Design review of the part built by this model. Coordinates are the model's own, in mm. Face numbers are marked on the shaded views. A direction names the side the tool comes from. Give positions to 0.01 mm unless a question says otherwise; leave off trailing zeros. Loops run counter-clockwise (first coordinate to the right, second up) from the corner with the lowest first, then second, coordinate; pieces in that order, holes last. Notation, with made-up numbers: (70, -1) -> (108, -1) arc R19 cw to (108, 34) -> close; hole circle Ø11 at (45, 60). An arc over 180 degrees is marked (long way). Use CSV: the item, a comma, the result in double quotes. Start each with the question number.
Item 1: We need section A-A (z = -52). State the section outline as (x, y) points, plus the area to 3 significant figures.
Item 2: Wall thickness on line 1 along Z through (x, y) = (23.5, -53); line 2 along Z through (x, y) = (13, 28.5); line 3 along Y through (x, z) = (16.75, -2.5): over which ranges is each line inside the solid? List them lowest first. Write a range as from..to.
Item 3: The part is to be moulded in two halves that separate along Z. For the marked faces 1, 2 and 3, say which applies: +Z half, -Z half, draft (parallel to the pull), parting line (faces both ways), or undercut.
Item 4: We need section B-B (y = 41.91). State the section outline as (x, z) points, plus the area to 3 significant figures.
Item 5: We need section D-D (x = 14.5). Count the separate pieces of the cut face and the enclosed holes in it, plus the area to 3 significant figures.
Item 6: We need section C-C (y = -29). State the section outline as (x, z) points, plus the area to 3 significant figures.
Item 7: Clearance check with flat-ended pins moving along their axes: pin 1 (5 mm diameter, centred on x = 8.5, y = 10, fed in from +Z); pin 2 (3 mm diameter, centred on y = -64.5, z = 6, fed in from -X); pin 3 (16.5 mm diameter, centred on y = -51.14, z = -30.23, fed in from +X); pin 4 (17 mm diameter, centred on y = -9.525, z = 0, fed in from +X). State where each tip first meets the part, or that it passes through.
Item 8: For the marked faces 4 and 5, list the 3-axis set-ups (+Z, -Z, +X, -X, +Y, -Y) from which the entire face can be reached by the end or side of a thin tool; tool diameter is ignored.
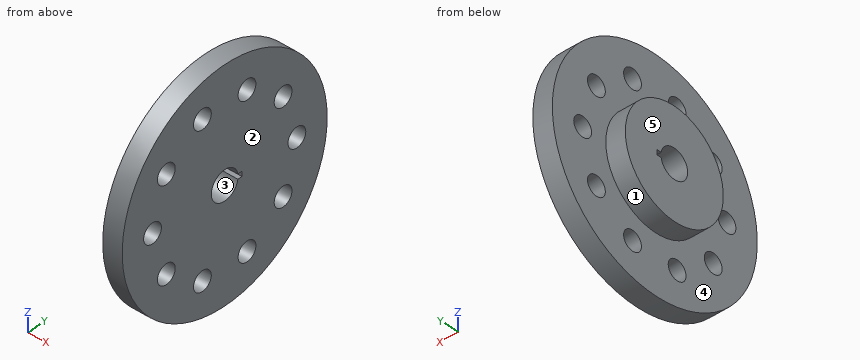
Autodesk Inventor part; units mm, degrees
ref_plane "YZ Plane" through (0, 0, 0) normal (1, 0, 0) x (0, 1, 0)
ref_plane "XZ Plane" through (0, 0, 0) normal (0, 1, 0) x (-1, 0, 0)
ref_plane "XY Plane" through (0, 0, 0) normal (0, 0, 1) x (1, 0, 0)
sketch "Sketch1" plane through (0, 0, 0) normal (0, 0, 1) x (1, 0, 0)
  line L0 (0, 0) -> (0, 25.4)
  line L1 (0, 25.4) -> (12.7, 25.4)
  line L2 (12.7, 25.4) -> (12.7, 63.5)
  line L3 (12.7, 63.5) -> (25.4, 63.5)
  line L4 (25.4, 63.5) -> (25.4, 0)
  line L5 (25.4, 0) -> (0, 0)
  line L6 (0, -9.525) -> (25.4, -9.525)
  dimension "d0" = 25.4
  dimension "d1" = 63.5
  dimension "d2" = 12.7
  dimension "d3" = 25.4
  dimension "d4" = 9.525
revolve "Revolution1" add sketch "Sketch1" angle 360 about axis through (0, -9.525, 0) along (1, 0, 0)
sketch "Sketch2" plane through (12.7, -9.525, 0) normal (-1, 0, 0) x (0, 0, 1)
  circle A0 centre (0, 0) radius 51.435 construction
  circle A1 centre (0, 0) radius 9.525
  circle A2 centre (0, 0) radius 73.025
  circle A3 centre (0, 0) radius 34.925
  point P0 (0, 9.525)
  point P1 (0, 51.435)
  point P2 (-30.2327, 41.6118)
  point P3 (-48.9176, 15.8943)
  point P4 (-48.9176, -15.8943)
  point P5 (-30.2327, -41.6118)
  point P6 (0, -51.435)
  point P7 (30.2327, -41.6118)
  point P8 (48.9176, -15.8943)
  point P9 (48.9176, 15.8943)
  point P10 (30.2327, 41.6118)
  dimension "d7" = 41.91
  dimension "d17" = 360
hole "Hole1" at (12.7, 41.91, 0) direction (1, 0, 0) diameter 12.7 end through all
hole "Hole2" at (12.7, 32.0868, -30.2327) at (12.7, 6.3693, -48.9176) at (12.7, -25.4193, -48.9176) at (12.7, -51.1368, -30.2327) at (12.7, -60.96, 0) at (12.7, -51.1368, 30.2327) at (12.7, -25.4193, 48.9176) at (12.7, 6.3693, 48.9176) at (12.7, 32.0868, 30.2327) direction (1, 0, 0) diameter 12.7 end through all
sketch "Sketch3" plane through (0, -9.525, 0) normal (-1, 0, 0) x (0, 0, 1)
  line L0 (-1.5875, 12.2962) -> (1.5875, 12.2962)
  line L1 (1.5875, 12.2962) -> (1.5875, 9.1212)
  line L2 (1.5875, 9.1212) -> (-1.5875, 9.1212)
  line L3 (-1.5875, 9.1212) -> (-1.5875, 12.2962)
  circle A0 centre (48.9176, 15.8943) radius 6.35
  circle A1 centre (0, 51.435) radius 6.35
  point P0 (0, 9.525)
  point P1 (0, 9.1212)
  point P2 (0, 12.2759)
  dimension "d26" = 3.175
  dimension "d27" = 3.175
  dimension "d29" = 1.5875
  dimension "d30" = 48.9176
  dimension "d31" = 0
  dimension "d33" = 42.3138
  dimension "d34" = 0
extrude "Extrusion1" cut sketch "Sketch3" against normal blind 50.8 contours L0 L1 L2 L3
properties part number "CircularPattern"
Results found:
1,outline,"(12.7, -60.8) -> (25.4, -60.8) -> (25.4, -30.97) -> (12.7, -30.97) -> close; (12.7, -19.87) -> (25.4, -19.87) -> (25.4, 0.82) -> (12.7, 0.82) -> close; (12.7, 11.92) -> (25.4, 11.92) -> (25.4, 41.75) -> (12.7, 41.75) -> close"
1,area,"1,020 mm²"
2,line 1,"-58.67..-36.3, -24.16..24.16, 36.3..58.67"
2,line 2,"-62.34..-35.47, -24.99..24.99, 35.47..62.34"
2,line 3,"-82.51..-66.8, -55.12..-18.72, -0.33..36.07, 47.75..63.46"
3,face 1,"parting line"
3,face 2,"draft"
3,face 3,"undercut"
4,outline,"(12.7, -51.84) -> (25.4, -51.84) -> (25.4, -6.35) -> (12.7, -6.35) -> close; (12.7, 6.35) -> (25.4, 6.35) -> (25.4, 51.84) -> (12.7, 51.84) -> close"
4,area,"1,160 mm²"
5,separate pieces,"1"
5,enclosed holes,"11"
5,area,"15,200 mm²"
6,outline,"(0, -28.99) -> (12.7, -28.99) -> (12.7, -43.67) -> (25.4, -43.67) -> (25.4, 43.67) -> (12.7, 43.67) -> (12.7, 28.99) -> (0, 28.99) -> close; (12.7, -70.38) -> (25.4, -70.38) -> (25.4, -54.16) -> (12.7, -54.16) -> close; (12.7, 54.16) -> (25.4, 54.16) -> (25.4, 70.38) -> (12.7, 70.38) -> close"
6,area,"2,260 mm²"
7,pin 1,"z = 30.49"
7,pin 2,"x = 12.7"
7,pin 3,"x = 25.4"
7,pin 4,"through"
8,face 4,"-X"
8,face 5,"+Z, -Z, -X, +Y, -Y"
